```python
from build123d import *

# Parameters (mm, degrees)
SKETCH1_R               = 1.25
BOSS_EXTRUDE1_DEPTH     = 8.3
SKETCH2_R               = 1.25
CUT_EXTRUDE1_DEPTH      = 3.700074126
CUT_EXTRUDE1_DEPTH_BACK = 8.770575704


with BuildPart() as part:
    # Sketch1 → Boss-Extrude1 (new body)
    with BuildSketch(Plane(origin=(0, 0, 0), x_dir=(1, 0, 0), z_dir=(0, 1, 0))):
        with BuildLine():
            Line((35.434172296, 1.287491613), (35.622727971, 1.3307936))
            ThreePointArc((35.622727971, 1.3307936), (36.223294794, 7.531563888), (32.32905872, 2.668935167))
            ThreePointArc((32.32905872, 2.668935167), (0.027157554, -0.697665471), (-32.309217612, 2.319893124))
            ThreePointArc((-32.309217612, 2.319893124), (-36.261610619, 7.13771657), (-35.575715837, 0.943979283))
            Line((-35.575715837, 0.943979283), (-35.413230424, 0.907951956))
            ThreePointArc((-35.413230424, 0.907951956), (0.030803418, -2.69767479), (35.434172296, 1.287491613))
        make_face()
        with Locations((-35, 4.142580739)):
            Circle(SKETCH1_R, mode=Mode.SUBTRACT)
        with Locations((35, 4.520575704)):
            Circle(SKETCH1_R, mode=Mode.SUBTRACT)
    extrude(amount=BOSS_EXTRUDE1_DEPTH)

    # Sketch2 → Cut-Extrude1 (cut, two sides)
    with BuildSketch(Plane.XY) as cut_extrude1_sk:
        with Locations((7.505235468, 4.15)):
            Circle(SKETCH2_R)
        with Locations((-7.494764532, 4.15)):
            Circle(SKETCH2_R)
    extrude(amount=CUT_EXTRUDE1_DEPTH, mode=Mode.SUBTRACT)
    extrude(cut_extrude1_sk.sketch, amount=-CUT_EXTRUDE1_DEPTH_BACK, mode=Mode.SUBTRACT)


solid = part.part
```
Work out the finished part from the listing and answer in its coordinate system (mm). Give positions to 0.01 mm unless a question says otherwise; leave off trailing zeros. Write each loop counter-clockwise with the first axis right and the second up, starting at its lowest first coordinate (ties: lowest second). Pieces come first, ordered by that corner, then holes. Notation, with made-up numbers: (-3.75, -35.5) -> (2.25, -35.5) arc R11 cw to (2.25, -21.5) -> close; hole circle Ø3 at (23, 58.5). An arc over 180 degrees is marked (long way). Write item = value, one per line.
Q1. Flat-ended cylindrical pins translate along their axes: pin 1 Ø2 at (y, z) = (4, -5.5) entering from -X; pin 2 Ø1.5 at (y, z) = (1.5, -1) entering from +X; pin 3 Ø1 at (y, z) = (5, -1.5) entering from -X. Find the tip coordinate at first contact, or state that the pin passes through.
Computed values:
pin_1 = -38.23
pin_2 = 36.7
pin_3 = -37.44
Q2. Section C-C on x = -2.5 is taken. Determine the outline of the cut face in (y, z).
Computed values:
outline = (0, 0.69) -> (8.3, 0.69) -> (8.3, 2.69) -> (0, 2.69) -> close
Q3. Section B-B on y = 1 is taken. Determine the outline of the cut face in (x, z).
Computed values:
outline = (-35.58, -0.94) arc R3.25 ccw (long way) to (-32.31, -2.32) arc R165.21 cw to (32.33, -2.67) arc R3.25 ccw (long way) to (35.62, -1.33) -> (35.43, -1.29) arc R167.21 ccw to (-35.41, -0.91) -> close; hole circle Ø2.5 at (-35, -4.14); hole circle Ø2.5 at (35, -4.52)
Q4. For a pull along Y with two mould halves and no side action, classify faces 1 (the cylindrical face through (8.698, 4.525, 1.47)), 2 (the flat face through (0, 0, 1)), 3 (the cylindrical face through (-35.92, 4.09, -4.99)) as pulls with the +Y half, pulls with the -Y half, needs draft (parallel to the pull), parting line crosses it, or undercut.
Computed values:
face_1 = undercut
face_2 = pulls with the -Y half
face_3 = needs draft
Q5. Section D-D on x = -25 is taken. Determine the outline of the cut face in (y, z), and give its area (3 significant figures).
Computed values:
outline = (0, -1.07) -> (8.3, -1.07) -> (8.3, 0.95) -> (0, 0.95) -> close
area = 16.8 mm^2
Q6. Section A-A on y = 4.15 is taken. Determine the outline of the cut face in (x, z), and give its area (3 significant figures).
Computed values:
outline = (-35.58, -0.94) arc R3.25 ccw (long way) to (-32.31, -2.32) arc R165.21 cw to (-8.74, 0.51) -> (-8.74, 2.51) arc R167.21 ccw to (-35.41, -0.91) -> close; (-6.24, 0.61) arc R165.21 cw to (6.26, 0.55) -> (6.26, 2.55) arc R167.21 ccw to (-6.24, 2.61) -> close; (8.76, 0.42) arc R165.21 cw to (32.33, -2.67) arc R3.25 ccw (long way) to (35.62, -1.33) -> (35.43, -1.29) arc R167.21 ccw to (8.76, 2.42) -> close; hole circle Ø2.5 at (-35, -4.14); hole circle Ø2.5 at (35, -4.52)
area = 181 mm^2
Q7. Consider line 1 along X through (y, z) = (2, -4.75); line 2 along Z through (x, y) = (-1, 5.5); line 3 along X through (y, z) = (0.75, -6.5). Determine where each line is inside the solid, lowest interval first.
Computed values:
line_1 = -38.19 to -36.09, -33.91 to -31.81, 31.76 to 33.77, 36.23 to 38.24
line_2 = 0.7 to 2.7
line_3 = -37.24 to -32.76, 32.42 to 37.58
